Autodesk Inventor part; units mm, degrees
ref_plane "YZ Plane" through (0, 0, 0) normal (1, 0, 0) x (0, 1, 0)
ref_plane "XZ Plane" through (0, 0, 0) normal (0, 1, 0) x (-1, 0, 0)
ref_plane "XY Plane" through (0, 0, 0) normal (0, 0, 1) x (1, 0, 0)
sketch "Sketch1" plane through (0, 0, 0) normal (0, 0, 1) x (1, 0, 0)
  line L0 (2.8868, 0) -> (1.4434, -2.5)
  line L1 (1.4434, -2.5) -> (-1.4434, -2.5)
  line L2 (-1.4434, -2.5) -> (-2.8868, 0)
  line L3 (-2.8868, 0) -> (-1.4434, 2.5)
  line L4 (-1.4434, 2.5) -> (1.4434, 2.5)
  line L5 (1.4434, 2.5) -> (2.8868, 0)
  point P0 (0, 0)
  point P1 (0, 0)
  dimension "d0" = 5
extrude "Extrusion1" add sketch "Sketch1" along normal blind 6
sketch "Sketch3" plane through (0, 0, 0) normal (0, 0, -1) x (-1, 0, 0)
  circle A0 centre (0, 0) radius 1.25
  dimension "d6" = 2.5
extrude "Extrusion3" cut sketch "Sketch3" against normal through all
sketch "Sketch4" plane through (0, 0, 6) normal (0, 0, 1) x (1, 0, 0)
  circle A0 centre (0, 0) radius 1.25
  dimension "d9" = 2.5
extrude "Extrusion4" add sketch "Sketch4" along normal blind 6
sketch "Sketch5" plane through (0, 0, 6) normal (0, 0, -1) x (-1, 0, 0)
  circle A0 centre (0, 0) radius 1.25
extrude "Extrusion5" add sketch "Sketch5" along normal blind 3
properties part number "M2.5x6mm_Standoff_ 971060151"
Read the model definition and answer for the solid it produces. Units are mm, in the model's axes. A direction names the side the tool comes from. Coordinates: 2 decimals unless noted, no trailing zeros. Write each loop counter-clockwise with the first axis right and the second up, starting at its lowest first coordinate (ties: lowest second). Pieces come first, ordered by that corner, then holes. Notation, with made-up numbers: M 80,16 L 126,16 A17 ccw 126,29 Z; hole C 63.25,-34 d11. An arc over 180 degrees is marked long. Use a Markdown table: item, result.
Q1. The part is cut by section B-B, the plane z = 3.5. Write down the section's boundary in (x, y).
Answer block:
| item | result |
|---|---|
| outline | M -2.89,0 L -1.44,-2.5 L 1.44,-2.5 L 2.89,0 L 1.44,2.5 L -1.44,2.5 Z |
Q2. Each of these flat-tipped pins is pushed along its axis until it touches: pin 1 Ø2.5 at (x, y) = (-1.5, -0.5) entering from +Z; pin 2 Ø1.5 at (x, y) = (-1.5, 1.5) entering from +Z; pin 3 Ø0.8 at (x, y) = (0, 0) entering from -Z. Where does it stop, or does it pass through?
Answer block:
| item | result |
|---|---|
| pin 1 | stops at z = 12 |
| pin 2 | stops at z = 6 |
| pin 3 | stops at z = 3 |
Q3. The part is cut by section A-A, the plane x = 0. Write down the section's boundary in (y, z).
Answer block:
| item | result |
|---|---|
| outline | M -2.5,0 L -1.25,0 L -1.25,3 L 1.25,3 L 1.25,0 L 2.5,0 L 2.5,6 L 1.25,6 L 1.25,12 L -1.25,12 L -1.25,6 L -2.5,6 Z |
Q4. The part is cut by section C-C, the plane y = -0.75. Write down the section's boundary in (x, z), then the cut area to 3 significant figures.
Answer block:
| item | result |
|---|---|
| outline | M -2.45,0 L -1,0 L -1,3 L 1,3 L 1,0 L 2.45,0 L 2.45,6 L 1,6 L 1,12 L -1,12 L -1,6 L -2.45,6 Z |
| area | 35.4 mm2 |
Q5. Which of the six approach directions +Z, -Z, +X, -X, +Y, -Y give full straight-line access (tool end or side, diameter ignored) to faces 1 (the face through (0, -2.5, 3)), 2 (the face through (-0.27, 1.22, 8.96)), 3 (the face through (0, 0, 3))?
Answer block:
| item | result |
|---|---|
| face 1 | +Z, -Z, +X, -X, -Y |
| face 2 | +Z |
| face 3 | -Z |
Q6. Straight lines are drawn through the part: L1, parallel to Y at x = 0, z = 2; L2, parallel to Z at x = 1.55, y = 0.1; L3, parallel to Z at x = -0.2, y = 0.35. For each, find the intervals that lie inside material, in ascending order. Write a range as [from, to].
Answer block:
| item | result |
|---|---|
| L1 | y = [-2.5, -1.25], [1.25, 2.5] |
| L2 | z = [0, 6] |
| L3 | z = [3, 12] |
Q7. The part is cut by section D-D, the plane z = 11. Write down the section's boundary in (x, y), then the cut area to 3 significant figures.
Answer block:
| item | result |
|---|---|
| outline | C 0,0 d2.5 |
| area | 4.91 mm2 |
Q8. Determine the mould class of faces 4 (the face through (1, 1, 6)), 5 (the face through (-2.175, 1.233, 2.958)), 6 (the face through (0.27, -1.22, 1.48)), 7 (the face through (2.175, -1.233, 2.958)) for opening direction Y: released by +Y, released by -Y, zero draft, split by the parting line, or undercut.
Answer block:
| item | result |
|---|---|
| face 4 | zero draft |
| face 5 | released by +Y |
| face 6 | undercut |
| face 7 | released by -Y |
